```python
from build123d import *

# Parameters (mm, degrees)
SKETCH2_W           = 30
SKETCH2_H           = 65
BOSS_EXTRUDE1_DEPTH = 10
BOSS_EXTRUDE2_DEPTH = 30
CUT_EXTRUDE1_DEPTH  = 65.031242374
SKETCH6_R           = 3.5
CUT_EXTRUDE2_DEPTH  = 65.031242374


with BuildPart() as part:
    # Sketch2 → Boss-Extrude1 (new body)
    with BuildSketch(Plane(origin=(0, 0, 0), x_dir=(1, 0, 0), z_dir=(0, 1, 0))):
        with Locations((15, 32.5)):
            Rectangle(SKETCH2_W, SKETCH2_H)
    extrude(amount=BOSS_EXTRUDE1_DEPTH)

    # Sketch4 → Boss-Extrude2 (add)
    with BuildSketch(Plane(origin=(30, 0, 0), x_dir=(0, 0, -1), z_dir=(1, 0, 0))):
        with BuildLine():
            Line((30, 10), (30, 40))
            Line((30, 40), (25, 40))
            Line((25, 40), (25, 13))
            ThreePointArc((25, 13), (24.121320344, 10.878679656), (22, 10))
            Line((22, 10), (30, 10))
        make_face()
        with BuildLine():
            Line((43, 10), (35, 10))
            Line((35, 10), (35, 40))
            Line((35, 40), (40, 40))
            Line((40, 40), (40, 13))
            ThreePointArc((40, 13), (40.878679656, 10.878679656), (43, 10))
        make_face()
    extrude(amount=-BOSS_EXTRUDE2_DEPTH)

    # Sketch5 → Cut-Extrude1 (cut, through all)
    with BuildSketch(Plane(origin=(0, 0, -40), x_dir=(-1, 0, 0), z_dir=(0, 0, -1))):
        with BuildLine():
            Line((0, 13), (0, 40))
            Line((0, 40), (0, 41.88167297))
            Line((0, 41.88167297), (-30, 41.88167297))
            Line((-30, 41.88167297), (-30, 40))
            Line((-30, 40), (-30, 13))
            Line((-30, 13), (-28.5, 26.5))
            ThreePointArc((-28.5, 26.5), (-15, 40), (-1.5, 26.5))
            Line((-1.5, 26.5), (0, 13))
        make_face()
    extrude(amount=-CUT_EXTRUDE1_DEPTH, mode=Mode.SUBTRACT)

    # Sketch6 → Cut-Extrude2 (cut, through all)
    with BuildSketch(Plane(origin=(0, 0, -40), x_dir=(-1, 0, 0), z_dir=(0, 0, -1))):
        with Locations((-15, 26.5)):
            Circle(SKETCH6_R)
    extrude(amount=-CUT_EXTRUDE2_DEPTH, mode=Mode.SUBTRACT)


solid = part.part
```
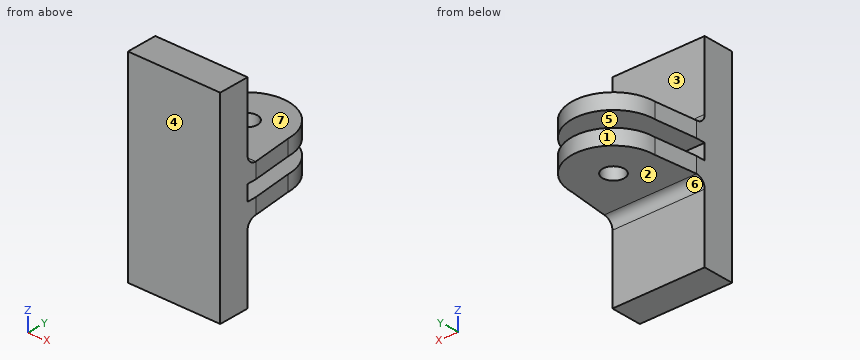
Check sheet for the modelled part. Datum: model origin and axes. Units: mm. Face numbers are marked on the shaded views. A direction names the side the tool comes from. Coordinates: 2 decimals unless noted, no trailing zeros. Loops run counter-clockwise (first coordinate to the right, second up) from the corner with the lowest first, then second, coordinate; pieces in that order, holes last. Notation, with made-up numbers: M 42.5,-21.5 L 89.5,-21.5 A7 ccw 89.5,-12.5 Z; hole C 11.5,18.5 d5. An arc over 180 degrees is marked long. Answer as a JSON object with one key per item and string values.
1. Scan lines: L1, parallel to Y at x = 15, z = -27.6; L2, parallel to Z at x = 25.5, y = 23; L3, parallel to Y at x = 18.5, z = -18. Record each from-to range of solid material in increasing order. Write a range as from..to.
Outcome:
{"L1": "0..23, 30..40", "L2": "-40..-35, -30..-25", "L3": "0..10"}
2. Sectioned sample at B-B on y = 20.5. Record the cut outline in (x, z).
Outcome:
{"outline": "M 0.83,-40 L 29.17,-40 L 29.17,-35 L 0.83,-35 Z; M 0.83,-30 L 29.17,-30 L 29.17,-25 L 0.83,-25 Z"}
3. Sectioned sample at C-C on x = 6.75. Record the cut outline in (y, z), and give its area (3 significant figures).
Outcome:
{"outline": "M 0,-65 L 10,-65 L 10,-43 A3 cw 13,-40 L 37.19,-40 L 37.19,-35 L 10,-35 L 10,-30 L 37.19,-30 L 37.19,-25 L 13,-25 A3 cw 10,-22 L 10,0 L 0,0 Z", "area": "926 mm²"}
4. Depth check by flat-ended pin: P1, Ø11, axis at x = 15, y = 26.5, coming from the +Z side; P2, Ø17.5, axis at x = 20.5, z = -15, coming from the +Y side; P3, Ø9, axis at x = 15, y = 26.5, coming from the -Z side; P4, Ø10, axis at y = 19.5, z = -18.5, coming from the -X side. Enter the tip coordinate at first touch or a pass-through.
Outcome:
{"P1": "z = -25", "P2": "y = 10.56", "P3": "z = -40", "P4": "through"}
5. Sectioned sample at A-A on x = 15. Record the cut outline in (y, z).
Outcome:
{"outline": "M 0,-65 L 10,-65 L 10,-43 A3 cw 13,-40 L 23,-40 L 23,-35 L 10,-35 L 10,-30 L 23,-30 L 23,-25 L 13,-25 A3 cw 10,-22 L 10,0 L 0,0 Z; M 30,-40 L 40,-40 L 40,-35 L 30,-35 Z; M 30,-30 L 40,-30 L 40,-25 L 30,-25 Z"}
6. Access from +Z, -Z, +X, -X, +Y, -Y to the whole of each face (thin tool, end or side, straight path). Record for the marked faces 1, 2 and 3.
Outcome:
{"face 1": "+Z, -Z, +Y", "face 2": "-Z, +X, -X, +Y", "face 3": "+Z, +X, -X, +Y"}
7. Release check for a two-part mould opening along Z. For the marked faces 4, 5, 6 and 7 record: pulls with the +Z half, pulls with the -Z half, needs draft (parallel to the pull), parting line crosses it, or undercut.
Outcome:
{"face 4": "needs draft", "face 5": "undercut", "face 6": "pulls with the -Z half", "face 7": "pulls with the +Z half"}
8. Sectioned sample at D-D on x = 10.75. Record the cut outline in (y, z).
Outcome:
{"outline": "M 0,-65 L 10,-65 L 10,-43 A3 cw 13,-40 L 39.31,-40 L 39.31,-35 L 10,-35 L 10,-30 L 39.31,-30 L 39.31,-25 L 13,-25 A3 cw 10,-22 L 10,0 L 0,0 Z"}
